Geometry check sheet. Reference: the model listing, model coordinates, mm. Face numbers are marked on the shaded views. A direction names the side the tool comes from. Coordinates: 2 decimals unless noted, no trailing zeros. Loops run counter-clockwise (first coordinate to the right, second up) from the corner with the lowest first, then second, coordinate; pieces in that order, holes last. Notation, with made-up numbers: M 6.25,35 L 64.25,35 A23 cw 64.25,69 Z; hole C 36.5,55 d8. An arc over 180 degrees is marked long. Use CSV: the item, a comma, the result in double quotes.
```python
from build123d import *

# Parameters (mm, degrees)
CROQUIS1_R              = 15
SALIENTE_EXTRUIR1_DEPTH = 40
CROQUIS2_R              = 20
SALIENTE_EXTRUIR2_DEPTH = 25
CROQUIS3_R              = 0.884543568
SALIENTE_EXTRUIR3_DEPTH = 3
CROQUIS4_R              = 5
CROQUIS4_R_2            = 2.5
SALIENTE_EXTRUIR4_DEPTH = 3
CORTAR_EXTRUIR1_DEPTH   = 3
REDONDEO3_R             = 1
CROQUIS6_R              = 2
CORTAR_EXTRUIR2_DEPTH   = 10


with BuildPart() as part:
    # Croquis1 → Saliente-Extruir1 (new body)
    with BuildSketch(Plane.XY):
        Circle(CROQUIS1_R)
    extrude(amount=SALIENTE_EXTRUIR1_DEPTH)

    # Croquis2 → Saliente-Extruir2 (add)
    with BuildSketch(Plane.XY.offset(40)):
        Circle(CROQUIS2_R)
    extrude(amount=SALIENTE_EXTRUIR2_DEPTH)

    # Croquis3 → Saliente-Extruir3 (add)
    with BuildSketch(Plane(origin=(0, 0, 0), x_dir=(-1, 0, 0), z_dir=(0, 0, -1))):
        with Locations(Location((0, 0, 0), (0, 0, 180))):
            Circle(CROQUIS3_R)
    extrude(amount=SALIENTE_EXTRUIR3_DEPTH)

    # Croquis4 → Saliente-Extruir4 (add)
    with BuildSketch(Plane.XY.offset(65)):
        with Locations((0, 12.5)):
            Circle(CROQUIS4_R)
        with Locations((0, 12.5)):
            Circle(CROQUIS4_R_2, mode=Mode.SUBTRACT)
    extrude(amount=SALIENTE_EXTRUIR4_DEPTH)

    # Croquis5 → Cortar-Extruir1 (cut)
    with BuildSketch(Plane(origin=(0, 0, 0), x_dir=(-1, 0, 0), z_dir=(0, 0, -1))):
        with BuildLine():
            Line((-3.149243081, 8.006162221), (-4.211738534, 10.70729095))
            ThreePointArc((-4.211738534, 10.70729095), (-9.509061365, 6.477852492), (-11.505860288, 0))
            Line((-11.505860288, 0), (-8.60327644, 0))
            ThreePointArc((-8.60327644, 0), (-7.110210064, 4.843684378), (-3.149243081, 8.006162221))
        make_face()
        with BuildLine():
            Line((-8.063121691, -3.000405654), (-10.783467475, -4.012686155))
            ThreePointArc((-10.783467475, -4.012686155), (-6.565645996, -9.44865671), (0, -11.505860288))
            Line((0, -11.505860288), (0, -8.60327644))
            ThreePointArc((0, -8.60327644), (-4.90933021, -7.065043693), (-8.063121691, -3.000405654))
        make_face()
        with BuildLine():
            ThreePointArc((8.60327644, 0), (7.097403678, -4.862430105), (3.106945666, -8.022671259))
            Line((3.106945666, -8.022671259), (4.012686155, -10.783467475))
            ThreePointArc((4.012686155, -10.783467475), (9.44865671, -6.565645996), (11.505860288, 0))
            Line((11.505860288, 0), (8.60327644, 0))
        make_face()
        with BuildLine():
            ThreePointArc((7.897835112, 3.411827377), (4.725646591, 7.189202306), (0, 8.60327644))
            Line((0, 8.60327644), (0, 11.505860288))
            ThreePointArc((0, 11.505860288), (6.319990974, 9.614704106), (10.562416308, 4.562913838))
            Line((10.562416308, 4.562913838), (7.897835112, 3.411827377))
        make_face()
    extrude(amount=-CORTAR_EXTRUIR1_DEPTH, mode=Mode.SUBTRACT)

    # Redondeo3
    redondeo3_edges = [part.edges().sort_by_distance(p)[0] for p in [
        (-15, 0, 0),
    ]]
    fillet(redondeo3_edges, radius=REDONDEO3_R)

    # Croquis6 → Cortar-Extruir2 (cut)
    with BuildSketch(Plane.XY.offset(65)):
        with Locations((15, 0)):
            Circle(CROQUIS6_R)
        with Locations((-15, 0)):
            Circle(CROQUIS6_R)
        with Locations((0, -15)):
            Circle(CROQUIS6_R)
    extrude(amount=-CORTAR_EXTRUIR2_DEPTH, mode=Mode.SUBTRACT)


solid = part.part
```
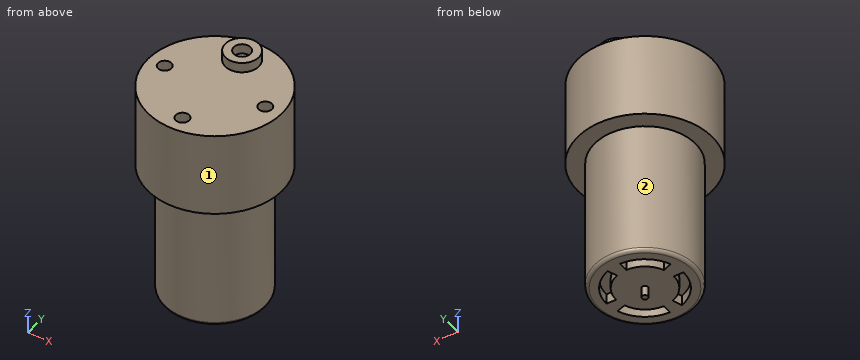
1. Set-up check for the marked faces 1 and 2: record each of +Z, -Z, +X, -X, +Y, -Y from which the full face is reachable in a straight line by a thin tool's end or side.
The answers:
face 1,"+Z, -Z"
face 2,"-Z"
2. Section check B-B, the plane z = 63. Record the cut outline in (x, y), plus the area to 3 significant figures.
The answers:
outline,"C 0,0 d40; hole C -15,0 d4; hole C 0,-15 d4; hole C 15,0 d4"
area,"1,220 mm^2"
3. Thickness scan on line 1 (Y direction, x = 0, z = 66.25); line 2 (Z direction, x = -3.5, y = 3); line 3 (Z direction, x = 13, y = -10.5). Record the ranges inside material, lowest first. Write a range as [from, to].
The answers:
line 1,"[7.5, 10], [15, 17.5]"
line 2,"[0, 65]"
line 3,"[40, 65]"
4. Section check C-C, the plane z = 49.5. Record the cut outline in (x, y).
The answers:
outline,"C 0,0 d40"
5. Section check A-A, the plane z = 12. Record the cut outline in (x, y), plus the area to 3 significant figures.
The answers:
outline,"C 0,0 d30"
area,"707 mm^2"
6. Gauge pin test, flat ends, axial feed: P1, Ø3, axis at x = 10, z = 1.5, coming from the +Y side; P2, Ø4.5, axis at x = -15, y = 0, coming from the +Z side; P3, Ø8, axis at y = -9.5, z = 24.5, coming from the -X side. Record the tip position at first contact, or that the pin passes through.
The answers:
P1,"y = 12.36"
P2,"z = 65"
P3,"x = -13.96"
